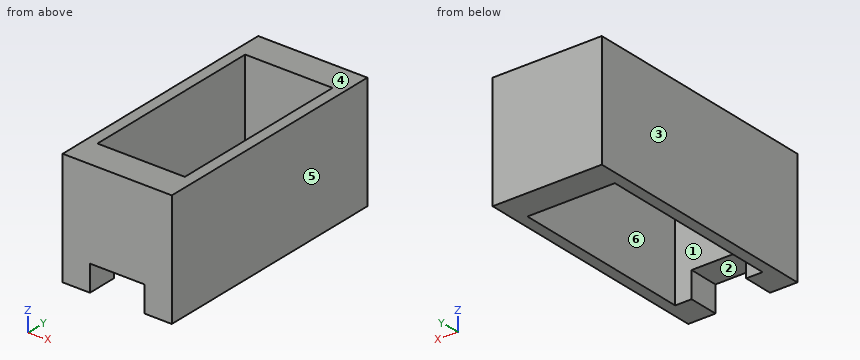
from build123d import *

# Parameters (mm, degrees)
SKETCH2_W           = 25.4
SKETCH2_H           = 57.15
SKETCH2_W_2         = 20.32
SKETCH2_H_2         = 43.18
BOSS_EXTRUDE2_DEPTH = 26.67
CUT_EXTRUDE1_REACH  = 59.15
SKETCH3_W           = 12.7
SKETCH3_H           = 12.7


with BuildPart() as part:
    # Sketch2 → Boss-Extrude2 (new body)
    with BuildSketch(Plane.XY):
        Rectangle(SKETCH2_W, SKETCH2_H)
        Rectangle(SKETCH2_W_2, SKETCH2_H_2, mode=Mode.SUBTRACT)
    extrude(amount=BOSS_EXTRUDE2_DEPTH)

    # Sketch3 → Cut-Extrude1 (cut, up to next)
    with BuildSketch(Plane.XZ.offset(28.575), mode=Mode.PRIVATE) as cut_extrude1_sk1:
        with Locations((0, -0.299628978)):
            Rectangle(SKETCH3_W, SKETCH3_H)
    cut_extrude1_tool1 = extrude(cut_extrude1_sk1.sketch, amount=-CUT_EXTRUDE1_REACH, mode=Mode.PRIVATE) & part.part
    add(cut_extrude1_tool1.solids().sort_by_distance((0, -28.575, -0.299629))[0], mode=Mode.SUBTRACT)


solid = part.part
The listing builds one solid part. Answer for the finished solid, in the listing's coordinates (mm). Face numbers are marked on the shaded views. A direction names the side the tool comes from. Coordinates: 2 decimals unless noted, no trailing zeros. Write each loop counter-clockwise with the first axis right and the second up, starting at its lowest first coordinate (ties: lowest second). Pieces come first, ordered by that corner, then holes. Notation, with made-up numbers: M 37,-39.5 L 52,-39.5 A34 cw 52,-0.5 Z; hole C -11,63.25 d1. An arc over 180 degrees is marked long. Put each result on its own line as item: value. Start each with the question number.
1. A cutting plane is placed at A-A on x = 5.5. Write down the section's boundary in (y, z) (3 decimals), then the cut area to 3 significant figures.
2. For a pull along X with two mould halves and no side action, classify the marked faces 4, 5 and 6 as pulls with the +X half, pulls with the -X half, needs draft (parallel to the pull), parting line crosses it, or undercut.
3. Consider line 1 (Y direction, x = -8, z = 16.75) (3 decimals); line 2 (X direction, y = 19, z = 8); line 3 (X direction, y = -24, z = 4.5). Determine where each line is inside the solid, lowest interval first. Write a range as from..to.
4. A cutting plane is placed at C-C on z = 23.5. Write down the section's boundary in (x, y) (3 decimals).
5. Which of the six approach directions +Z, -Z, +X, -X, +Y, -Y give full straight-line access (tool end or side, diameter ignored) to the marked faces 1, 2 and 3?
6. Flat-ended cylindrical pins translate along their axes: P1, Ø10, axis at x = 7.5, y = 3, coming from the +Z side; P2, Ø7.5, axis at x = -1, y = -24, coming from the -Z side. Find the tip coordinate at first contact, or state that the pin passes through.
7. A cutting plane is placed at B-B on y = 6. Write down the section's boundary in (x, z), then the cut area to 3 significant figures.
Resolved:
1. outline: M -28.575,6.05 L -21.59,6.05 L -21.59,26.67 L -28.575,26.67 Z; M 21.59,0 L 28.575,0 L 28.575,26.67 L 21.59,26.67 Z
1. area: 330 mm2
2. face 4: needs draft
2. face 5: pulls with the +X half
2. face 6: undercut
3. line 1: y = -28.575..-21.59, 21.59..28.575
3. line 2: x = -12.7..-10.16, 10.16..12.7
3. line 3: x = -12.7..-6.35, 6.35..12.7
4. outline: M -12.7,-28.575 L 12.7,-28.575 L 12.7,28.575 L -12.7,28.575 Z; hole M -10.16,-21.59 L 10.16,-21.59 L 10.16,21.59 L -10.16,21.59 Z
5. face 1: +Z, -Z
5. face 2: -Z, -Y
5. face 3: +Z, -Z, -X, +Y, -Y
6. P1: stops at z = 26.67
6. P2: stops at z = 6.05
7. outline: M -12.7,0 L -10.16,0 L -10.16,26.67 L -12.7,26.67 Z; M 10.16,0 L 12.7,0 L 12.7,26.67 L 10.16,26.67 Z
7. area: 135 mm2
